Read the model definition and answer for the solid it produces. Units are mm, in the model's axes. A direction names the side the tool comes from. Coordinates: 2 decimals unless noted, no trailing zeros. Loops run counter-clockwise (first coordinate to the right, second up) from the corner with the lowest first, then second, coordinate; pieces in that order, holes last. Notation, with made-up numbers: (-32.75, 47.5) - (-0.75, 47.5) arc R30 cw to (-0.75, 72.5) - close; hole circle Ø9 at (48.5, 15.5). An arc over 180 degrees is marked (long way). Use one line per item in the form item = value. Start each with the question number.
1) A cutting plane is placed at C-C (x = 15). Give the vertices of the cut face in (y, z) (3 decimals).
2) Consider line 1 (Y direction, x = 0, z = 3.75) (3 decimals); line 2 (Z direction, x = 20, y = -20); line 3 (Y direction, x = 18, z = 135). Determine where each line is inside the solid, lowest interval first.
3) A cutting plane is placed at B-B (x = -4). State how many separate pieces and enclosed holes the cut face has, and give its area (3 significant figures).
4) Each of these flat-tipped pins is pushed along its axis until it touches: P1, Ø8, axis at x = 23.5, y = -23, coming from the -Z side; P2, Ø5, axis at x = 10, y = 7, coming from the +Z side; P3, Ø8.5, axis at x = 0, y = 0, coming from the -Z side. Where does it stop, or does it pass through?
5) A cutting plane is placed at A-A (z = 104). Give the vertices of the cut face in (x, y).
6) Which of the six approach directions +Z, -Z, +X, -X, +Y, -Y give full straight-line access (tool end or side, diameter ignored) to faces 1 (the face through (-0.909, 6.926, 3.131)), 2 (the face through (6.72, -6.826, 161.881)), 3 (the face through (18, 1.27, 162))?
7) A cutting plane is placed at D-D (z = 27). Give the vertices of the cut face in (x, y) (3 decimals).
8) The mould has two halves that part along X. Classify faces 4 (the face through (0, -30.48, 94)), 5 (the face through (0, 19.685, 178)), 6 (the face through (-30.48, 0, 94)): released by +X, released by -X, zero draft, split by the parting line, or undercut.
from build123d import *
from build123d.topology import SkipClean

# Parameters (mm, degrees)
SKETCH1_R           = 29.845
SKETCH1_R_2         = 26.67
BOSS_EXTRUDE1_DEPTH = 165.1
SKETCH2_W           = 59.69
SKETCH2_H           = 38.1
CUT_EXTRUDE1_DEPTH  = 171.409677102
BOSS_EXTRUDE2_DEPTH = 6.35
SKETCH5_R           = 29.845
SKETCH5_R_2         = 6.985
BOSS_EXTRUDE4_DEPTH = 6.35
BOSS_EXTRUDE5_START = -6.35
SKETCH4_R           = 29.845
SKETCH4_R_2         = 26.67
SKETCH4_R_3         = 6.985
BOSS_EXTRUDE5_DEPTH = 6.35
SKETCH6_W           = 60.96
SKETCH6_H           = 60.96
SKETCH6_R           = 29.845
BOSS_EXTRUDE7_DEPTH = 190.5
BOSS_EXTRUDE8_START = -25.4
SKETCH7_W           = 60.96
SKETCH7_H           = 60.96
SKETCH7_R           = 29.845
SKETCH7_W_2         = 39.37
SKETCH7_H_2         = 39.37
BOSS_EXTRUDE8_DEPTH = 25.4
SKETCH8_W           = 47.836836
SKETCH8_H           = 47.836836
SKETCH8_W_2         = 43.603672
SKETCH8_H_2         = 43.603672
CUT_EXTRUDE2_DEPTH  = 12.7
FILLET1_R           = 2.54
FILLET2_R           = 12.7


with BuildPart() as part:
    # Sketch1 → Boss-Extrude1 (new body)
    with BuildSketch(Plane.XY):
        Circle(SKETCH1_R)
        Circle(SKETCH1_R_2, mode=Mode.SUBTRACT)
    extrude(amount=BOSS_EXTRUDE1_DEPTH)

    # Sketch2 → Cut-Extrude1 (cut, through all)
    with BuildSketch(Plane(origin=(0, 0, 0), x_dir=(1, 0, 0), z_dir=(0, 1, 0))):
        with Locations((0, -18.194460122)):
            Rectangle(SKETCH2_W, SKETCH2_H)
    extrude(amount=-CUT_EXTRUDE1_DEPTH, mode=Mode.SUBTRACT)

    # Sketch3 → Boss-Extrude2 (add)
    with BuildSketch(Plane(origin=(0, 0, 0), x_dir=(-1, 0, 0), z_dir=(0, 0, -1))):
        with BuildLine():
            Line((-29.845, 0), (-6.985, 0))
            ThreePointArc((-6.985, 0), (0, 6.985), (6.985, 0))
            Line((6.985, 0), (29.845, 0))
            ThreePointArc((29.845, 0), (0, 29.845), (-29.845, 0))
        make_face()
    extrude(amount=-BOSS_EXTRUDE2_DEPTH)

    # Sketch5 → Boss-Extrude4 (add)
    with SkipClean():  # the faces are left unmerged after this step: merging them gives an invalid solid
        with BuildSketch(Plane(origin=(0, 0, 0), x_dir=(-1, 0, 0), z_dir=(0, 0, -1))):
            with Locations(Location((0, 0, 0), (0, 0, 180))):
                Circle(SKETCH5_R)
            with BuildLine():
                Line((26.639744744, 1.27), (9.33422749, 1.465384615))
                ThreePointArc((9.33422749, 1.465384615), (6.689709997, 6.703146826), (1.477288556, 9.397267918))
                Line((1.477288556, 9.397267918), (1.27, 26.639744744))
                ThreePointArc((1.27, 26.639744744), (18.858537854, 18.858537854), (26.639744744, 1.27))
            make_face(mode=Mode.SUBTRACT)
            with BuildLine():
                Line((-1.27, 26.639744744), (-1.27, 9.45004085))
                ThreePointArc((-1.27, 9.45004085), (-6.784923303, 6.762723487), (-9.517329266, 1.27))
                Line((-9.517329266, 1.27), (-26.639744744, 1.27))
                ThreePointArc((-26.639744744, 1.27), (-18.858537854, 18.858537854), (-1.27, 26.639744744))
            make_face(mode=Mode.SUBTRACT)
            Circle(SKETCH5_R_2, mode=Mode.SUBTRACT)
        extrude(amount=-BOSS_EXTRUDE4_DEPTH)

    # Sketch4 → Boss-Extrude5 (add)
    # profile 1 of 2: a face of its own
    with SkipClean():  # the faces are left unmerged after this step: merging them gives an invalid solid
        with BuildSketch(Plane.XY.offset(165.1).offset(BOSS_EXTRUDE5_START)):
            Circle(SKETCH4_R)
            with Locations(Location((0, 0, 0), (0, 0, 180))):
                Circle(SKETCH4_R_2, mode=Mode.SUBTRACT)
        # profile 2 of 2: a face of its own
        with BuildSketch(Plane.XY.offset(165.1).offset(BOSS_EXTRUDE5_START)):
            with BuildLine():
                Line((1.27, 9.45004085), (1.27, 26.639744744))
                ThreePointArc((1.27, 26.639744744), (0, 26.67), (-1.27, 26.639744744))
                Line((-1.27, 26.639744744), (-1.477288556, 9.397267918))
                ThreePointArc((-1.477288556, 9.397267918), (-6.689709997, 6.703146826), (-9.33422749, 1.465384615))
                Line((-9.33422749, 1.465384615), (-26.639744744, 1.27))
                ThreePointArc((-26.639744744, 1.27), (-26.67, 0), (-26.639744744, -1.27))
                Line((-26.639744744, -1.27), (-9.33422749, -1.465384615))
                ThreePointArc((-9.33422749, -1.465384615), (-6.689709997, -6.703146826), (-1.477288556, -9.397267918))
                Line((-1.477288556, -9.397267918), (-1.27, -26.639744744))
                ThreePointArc((-1.27, -26.639744744), (0, -26.67), (1.27, -26.639744744))
                Line((1.27, -26.639744744), (1.453480675, -9.425070814))
                ThreePointArc((1.453480675, -9.425070814), (6.780569847, -6.767038646), (9.488978712, -1.465384615))
                Line((9.488978712, -1.465384615), (26.639744744, -1.27))
                ThreePointArc((26.639744744, -1.27), (26.662435113, -0.635180167), (26.67, 0))
                ThreePointArc((26.67, 0), (26.662435113, 0.635180167), (26.639744744, 1.27))
                Line((26.639744744, 1.27), (9.517329266, 1.27))
                ThreePointArc((9.517329266, 1.27), (6.784923303, 6.762723487), (1.27, 9.45004085))
            make_face()
            with Locations(Location((0, 0, 0), (0, 0, 180))):
                Circle(SKETCH4_R_3, mode=Mode.SUBTRACT)
        extrude(amount=BOSS_EXTRUDE5_DEPTH)

    # Sketch6 → Boss-Extrude7 (add)
    with BuildSketch(Plane.XY):
        Rectangle(SKETCH6_W, SKETCH6_H)
        Circle(SKETCH6_R, mode=Mode.SUBTRACT)
    extrude(amount=BOSS_EXTRUDE7_DEPTH)

    # Sketch7 → Boss-Extrude8 (add)
    # profile 1 of 2: a face of its own
    with BuildSketch(Plane.XY.offset(190.5).offset(BOSS_EXTRUDE8_START)):
        Rectangle(SKETCH7_W, SKETCH7_H)
        Circle(SKETCH7_R, mode=Mode.SUBTRACT)
    # profile 2 of 2: a face of its own
    with BuildSketch(Plane.XY.offset(190.5).offset(BOSS_EXTRUDE8_START)):
        Circle(SKETCH7_R)
        Rectangle(SKETCH7_W_2, SKETCH7_H_2, mode=Mode.SUBTRACT)
    extrude(amount=BOSS_EXTRUDE8_DEPTH)

    # Sketch8 → Cut-Extrude2 (cut)
    with BuildSketch(Plane.XY.offset(190.5)):
        Rectangle(SKETCH8_W, SKETCH8_H)
        Rectangle(SKETCH8_W_2, SKETCH8_H_2, mode=Mode.SUBTRACT)
    extrude(amount=-CUT_EXTRUDE2_DEPTH, mode=Mode.SUBTRACT)

    # Fillet1
    # the kernel refuses this fillet: 2.54 mm, written as the material it adds along each edge
    with BuildSketch(Plane(origin=(19.685, -19.685, 165.1), x_dir=(-1, 0, 0), z_dir=(0, 0, 1)), Plane(origin=(19.685, 19.685, 165.1), x_dir=(0, -1, 0), z_dir=(0, 0, 1)), Plane(origin=(-19.685, -19.685, 165.1), x_dir=(0, 1, 0), z_dir=(0, 0, 1))) as fillet1_piece_1:
        with BuildLine():
            CenterArc((FILLET1_R, -FILLET1_R), FILLET1_R, 90, 90)
            Line((0, -FILLET1_R), (0, 0))
            Line((0, 0), (FILLET1_R, 0))
        make_face()
    extrude(amount=25.4)
    with BuildSketch(Plane(origin=(-19.685, 19.685, 165.1), x_dir=(0, -1, 0), z_dir=(0, 0, 1))) as fillet1_piece_2:
        with BuildLine():
            CenterArc((FILLET1_R, FILLET1_R), FILLET1_R, 180, 90)
            Line((0, FILLET1_R), (0, 0))
            Line((0, 0), (FILLET1_R, 0))
        make_face()
    extrude(amount=25.4)

    # Fillet2
    fillet2_edges = [part.edges().sort_by_distance(p)[0] for p in [
        (-30.48, 30.48, 95.25),
        (-30.48, -30.48, 95.25),
        (30.48, -30.48, 95.25),
        (30.48, 30.48, 95.25),
    ]]
    fillet(fillet2_edges, radius=FILLET2_R)


solid = part.part
Found:
q1.outline = (-30.48, 0) - (30.48, 0) - (30.48, 190.5) - (23.918, 190.5) - (23.918, 177.8) - (21.802, 177.8) - (21.802, 190.5) - (19.685, 190.5) - (19.685, 165.1) - (22.052, 165.1) - (22.052, 6.35) - (-25.802, 6.35) - (-25.802, 37.244) - (-22.052, 37.244) - (-22.052, 165.1) - (-19.685, 165.1) - (-19.685, 190.5) - (-21.802, 190.5) - (-21.802, 177.8) - (-23.918, 177.8) - (-23.918, 190.5) - (-30.48, 190.5) - close; (-1.403, 158.75) - (1.27, 158.75) - (1.27, 165.1) - (-1.403, 165.1) - close
q2.line_1 = -30.48 to -6.985, 6.985 to 30.48
q2.line_2 = 0 to 6.35, 37.24 to 190.5
q2.line_3 = -30.48 to -19.68, 19.68 to 30.48
q3.separate_pieces = 4
q3.enclosed_holes = 0
q3.area = 2,050 mm^2
q4.P1 = 0
q4.P2 = 6.35
q4.P3 = through
q5.outline = (-30.48, -17.78) arc R12.7 ccw to (-17.78, -30.48) - (17.78, -30.48) arc R12.7 ccw to (30.48, -17.78) - (30.48, 17.78) arc R12.7 ccw to (17.78, 30.48) - (-17.78, 30.48) arc R12.7 ccw to (-30.48, 17.78) - close; hole circle Ø53.34 at (0, 0)
q6.face_1 = +Z, -Z
q6.face_2 = +Z
q6.face_3 = none
q7.outline = (-30.48, -17.78) arc R12.7 ccw to (-17.78, -30.48) - (17.78, -30.48) arc R12.7 ccw to (30.48, -17.78) - (30.48, 17.78) arc R12.7 ccw to (17.78, 30.48) - (-17.78, 30.48) arc R12.7 ccw to (-30.48, 17.78) - close; hole (-29.845, 0) arc R29.845 ccw to (29.845, 0) - (26.67, 0) arc R26.67 ccw to (-26.67, 0) - close
q8.face_4 = zero draft
q8.face_5 = undercut
q8.face_6 = released by -X
